Here's how the part is built. I have some questions about the finished solid (model axes, mm). Face numbers are marked on the shaded views. Round coordinates to 2 decimals unless told otherwise and drop trailing zeros. Loops run counter-clockwise (first coordinate to the right, second up) from the corner with the lowest first, then second, coordinate; pieces in that order, holes last. Notation, with made-up numbers: (-18.75, -18) -> (-2.75, -18) arc R26 cw to (-2.75, -2) -> close; hole circle Ø11 at (88, 69.25). An arc over 180 degrees is marked (long way). One line per item, written item: value. Start each with the question number.
```python
from build123d import *

# Parameters (mm, degrees)
F0_R     = 36.718352
F1_DEPTH = 127
F3_R     = 38.474743
F4_DEPTH = 62.738
F6_D     = 6.35


with BuildPart() as f1:
    # F0 (on Front) → F1 (new body)
    with BuildSketch(Plane.XZ):
        Circle(F0_R)
    extrude(amount=F1_DEPTH)

    # F3 (on offset) → F4 (cut)
    with BuildSketch(Plane.XZ.offset(101.6)):
        with Locations((65.835573, 16.081614)):
            Circle(F3_R)
    extrude(amount=F4_DEPTH, mode=Mode.SUBTRACT)

    # F6 (through all)
    with Locations(Plane.XZ.offset(127)):
        with Locations((-18.136533, 9.744127), (0, 0)):
            Hole(F6_D / 2)


solid = f1.part
```
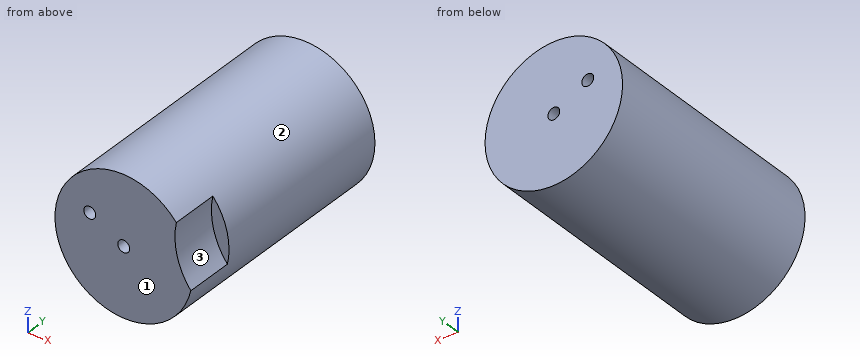
Q1. I want a section at D-D on y = -91.5. Please give me the cut outline in (x, z) (3 decimals).
Q2. If we mould it in two halves opening along Z, with no side actions, what happens to the marked faces 1, 2 and 3? For each: released by +Z, released by -Z, zero draft, split by the parting line, or undercut.
Q3. I want a section at C-C on x = 0. Please give me the cut outline in (y, z) (3 decimals), plus the area to 3 significant figures.
Q4. I want a section at B-B on z = 0. Please give me the cut outline in (x, y) (3 decimals).
Q5. If I drill on line 1 along Y through (x, z) = (29, 14.5); line 2 along X through (y, z) = (-36, 24.5); line 3 along X through (y, z) = (-60, 20), over which ranges is the centre line in solid material (lowest first)?
Q6. I want a section at A-A on x = -17.5. Please give me the cut outline in (y, z).
Q7. Will these pins go through, and if not, where does the flat tip stop? P1, Ø4, axis at x = 15.5, y = -54, coming from the +Z side; P2, Ø1.5, axis at x = 16.5, y = -112, coming from the +Z side; P3, Ø10, axis at x = -17, y = -105.5, coming from the +Z side; P4, Ø7.5, axis at x = 33, z = 3, coming from the -Y side.
Answers below:
1. outline: circle Ø73.437 at (0, 0); hole circle Ø6.35 at (-18.137, 9.744); hole circle Ø6.35 at (0, 0)
2. face 1: zero draft
2. face 2: split by the parting line
2. face 3: undercut
3. outline: (-127, -36.718) -> (0, -36.718) -> (0, -3.175) -> (-127, -3.175) -> close; (-127, 3.175) -> (0, 3.175) -> (0, 36.718) -> (-127, 36.718) -> close
3. area: 8,520 mm^2
4. outline: (-36.718, -127) -> (-3.175, -127) -> (-3.175, 0) -> (-36.718, 0) -> close; (3.175, -127) -> (30.883, -127) -> (30.883, -101.6) -> (36.718, -101.6) -> (36.718, 0) -> (3.175, 0) -> close
5. line 1: y = -101.6 to 0
5. line 2: x = -27.35 to 27.35
5. line 3: x = -30.79 to 30.79
6. outline: (-127, -32.28) -> (0, -32.28) -> (0, 6.63) -> (-127, 6.63) -> close; (-127, 12.85) -> (0, 12.85) -> (0, 32.28) -> (-127, 32.28) -> close
7. P1: stops at z = 34.15
7. P2: stops at z = 33.17
7. P3: stops at z = 34.7
7. P4: stops at y = -127
